```python
from build123d import *

# Parameters (mm, degrees)
F1_DEPTH   = 42
F3_SIZE2   = 25
F3_SIZE    = 20
F3_2_SIZE2 = 25
F3_2_SIZE  = 20
F4_D       = 20
F4_DEPTH   = 20.6886382592


with BuildPart() as f1:
    # F0 (on Front) → F1 (new body)
    with BuildSketch(Plane.XZ):
        Polygon((-20.6876382592, 40), (-20.6876382592, 0), (20.6876382592, 0), (20.6876382592, 40), (10.6876382592, 40), (10.6876382592, 10), (-10.6876382592, 10), (-10.6876382592, 40), align=None)
    extrude(amount=-F1_DEPTH)

    # F3
    f3_edges = [f1.edges().sort_by_distance(p)[0] for p in [
        (-15.687638, 0, 40),
    ]]
    f3_side = f1.faces().sort_by_distance((-15.687638, 21, 40))[0]
    chamfer(f3_edges, length=F3_SIZE, length2=F3_SIZE2, reference=f3_side)

    # F3#2
    f3_2_edges = [f1.edges().sort_by_distance(p)[0] for p in [
        (15.687638, 0, 40),
    ]]
    f3_2_side = f1.faces().sort_by_distance((15.687638, 21, 40))[0]
    chamfer(f3_2_edges, length=F3_2_SIZE, length2=F3_2_SIZE2, reference=f3_2_side)

    # F4 (through all, one way)
    with BuildSketch(Plane(origin=(0, 0, 0), x_dir=(0, 1, 0), z_dir=(-1, 0, 0))):
        with Locations((27.1959491074, -24.8310826719)):
            Circle(F4_D / 2)
    extrude(amount=-F4_DEPTH, mode=Mode.SUBTRACT)


solid = f1.part
```
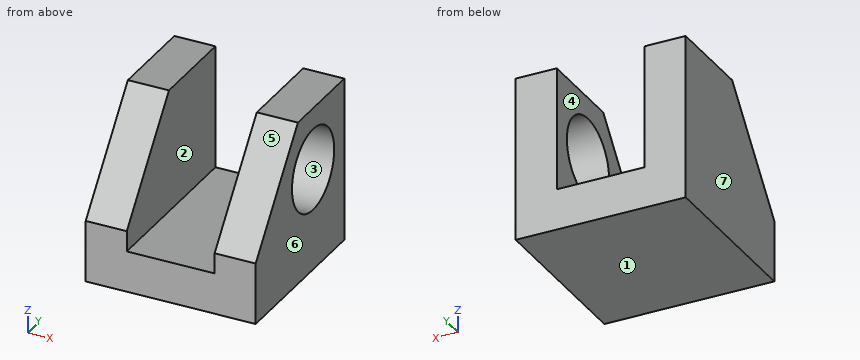
The model under review builds one solid part; all positions refer to its coordinate system, in mm. Face numbers are marked on the shaded views. A direction names the side the tool comes from. Round coordinates to 2 decimals unless told otherwise and drop trailing zeros. Loops run counter-clockwise (first coordinate to the right, second up) from the corner with the lowest first, then second, coordinate; pieces in that order, holes last.
Item 1: Clearance check with a flat-ended pin moving along its axis: pin 1 Ø3 at (x, y) = (9, 11) entering from +Z. State where the tip first meets the part, or that it passes through.
Determined:
pin 1: stops at z = 10
Item 2: Take a section at D-D (x = -16.5). Write out the cut boundary in (y, z), then the cut area to 3 significant figures.
Determined:
outline: (0, 0) - (42, 0) - (42, 40) - (20, 40) - (0, 15) - close
area: 1,430 mm2
Item 3: For the marked faces 1, 2 and 3, list the 3-axis set-ups (+Z, -Z, +X, -X, +Y, -Y) from which the entire face can be reached by the end or side of a thin tool; tool diameter is ignored.
Determined:
face 1: -Z, +X, -X, +Y, -Y
face 2: +Z, +Y, -Y
face 3: +X
Item 4: Take a section at A-A (z = 36). Write out the cut boundary in (x, y).
Determined:
outline: (-20.69, 16.8) - (-10.69, 16.8) - (-10.69, 42) - (-20.69, 42) - close; (10.69, 16.8) - (20.69, 16.8) - (20.69, 42) - (10.69, 42) - close
Item 5: Mouldability with a two-part tool opening along X and no side actions: class the marked faces 4, 5, 6 and 7 as released by +X, released by -X, zero draft, split by the parting line, or undercut.
Determined:
face 4: undercut
face 5: zero draft
face 6: released by +X
face 7: released by -X
Item 6: Take a section at B-B (y = 31). Write out the cut boundary in (x, z).
Determined:
outline: (-20.69, 0) - (20.69, 0) - (20.69, 15.58) - (10.69, 15.58) - (10.69, 10) - (-10.69, 10) - (-10.69, 40) - (-20.69, 40) - close; (10.69, 34.08) - (20.69, 34.08) - (20.69, 40) - (10.69, 40) - close
Item 7: Take a section at C-C (z = 31.5). Write out the cut boundary in (x, y).
Determined:
outline: (-20.69, 13.2) - (-10.69, 13.2) - (-10.69, 42) - (-20.69, 42) - close; (10.69, 13.2) - (20.69, 13.2) - (20.69, 19.74) - (10.69, 19.74) - close; (10.69, 34.65) - (20.69, 34.65) - (20.69, 42) - (10.69, 42) - close
Item 8: For line 1 (X direction, y = 5.5, z = 18.5); line 2 (X direction, y = 22, z = 23.5); line 3 (Z direction, x = 2.5, y = 36), list the stretches that pass through material, from the lowest coordinate up.
Determined:
line 1: x = -20.69 to -10.69, 10.69 to 20.69
line 2: x = -20.69 to -10.69
line 3: z = 0 to 10
